from build123d import *

# Parameters (mm, degrees)
BOSS_EXTRUDE1_DEPTH = 9
SKETCH2_R           = 2.165
CUT_EXTRUDE1_DEPTH  = 32.81587654


with BuildPart() as part:
    # Sketch1 → Boss-Extrude1 (new body)
    with BuildSketch(Plane.XY):
        with BuildLine():
            Line((29, -13.075), (29, -9.075))
            Line((29, -9.075), (13.955285737, -9.075))
            ThreePointArc((13.955285737, -9.075), (0, 0.425), (-13.955285737, -9.075))
            Line((-13.955285737, -9.075), (-29, -9.075))
            Line((-29, -9.075), (-29, -13.075))
            Line((-29, -13.075), (-10.897247359, -13.075))
            ThreePointArc((-10.897247359, -13.075), (0, -3.575), (10.897247359, -13.075))
            Line((10.897247359, -13.075), (29, -13.075))
        make_face()
    extrude(amount=BOSS_EXTRUDE1_DEPTH)

    # Sketch2 → Cut-Extrude1 (cut, through all)
    with BuildSketch(Plane(origin=(0, -9.075, 0), x_dir=(1, 0, 0), z_dir=(0, 1, 0))):
        with Locations(Location((-23.50000005, -4.5, 0), (0, 0, 180))):
            Circle(SKETCH2_R)
        with Locations(Location((23.50000005, -4.5, 0), (0, 0, 180))):
            Circle(SKETCH2_R)
    extrude(amount=-CUT_EXTRUDE1_DEPTH, mode=Mode.SUBTRACT)


solid = part.part
Read the model definition and answer for the solid it produces. Units are mm, in the model's axes. A direction names the side the tool comes from. Coordinates: 2 decimals unless noted, no trailing zeros. Loops run counter-clockwise (first coordinate to the right, second up) from the corner with the lowest first, then second, coordinate; pieces in that order, holes last. Notation, with made-up numbers: (69.5, 38) -> (110.5, 38) arc R16 cw to (110.5, 42) -> close; hole circle Ø5 at (1, -21.75). An arc over 180 degrees is marked (long way). Write item = value, one per line. Start each with the question number.
1) Given P1, Ø4.5, axis at x = 23, z = 5.5, coming from the +Y side (3 decimals); P2, Ø2, axis at x = -1.5, z = 7, coming from the -Y side; P3, Ø5, axis at x = 2, z = 6, coming from the +Y side (3 decimals); P4, Ø1.5, axis at x = -17.5, y = -8, coming from the -Z side, each flat-ended and moving along its own axis, determine where each tip first touches the part or whether it passes through.
2) The part is cut by section A-A, the plane z = 4.5. Determine the outline of the cut face in (x, y) (3 decimals).
3) The part is cut by section C-C, the plane y = -11. Determine the outline of the cut face in (x, z) (3 decimals).
4) For faces 1 (the face through (-20, -13.075, 4)), 2 (the face through (20, -9.075, 4)), 3 (the face through (-21, -9.075, 5)), determine the directions among +Z, -Z, +X, -X, +Y, -Y from which every point of the face is accessible in a straight line to the end or side of a thin tool.
5) Find the intervals of material crossed by L1, parallel to Z at x = -23.5, y = -10.65 (3 decimals); L2, parallel to Y at x = -14, z = 5.5 (3 decimals); L3, parallel to X at y = -6.5, z = 3.25, in increasing order. Write a range as from..to.
6) The part is cut by section B-B, the plane x = -23.5. Determine the outline of the cut face in (y, z) (3 decimals), plus the area to 3 significant figures.
7) The mould has two halves that part along X. Classify faces 4 (the face through (25.663, -11.047, 4.595)), 5 (the face through (0, -3, 0)), 6 (the face through (-21.337, -11.047, 4.595)), 7 (the face through (0.251, 0.423, 4.437)): pulls with the +X half, pulls with the -X half, needs draft (parallel to the pull), parting line crosses it, or undercut.
8) The part is cut by section D-D, the plane z = 8.25. Determine the outline of the cut face in (x, y) (3 decimals), plus the area to 3 significant figures.
Result:
q1.P1 = -9.075
q1.P2 = -3.86
q1.P3 = 0.425
q1.P4 = through
q2.outline = (-29, -13.075) -> (-25.665, -13.075) -> (-25.665, -9.075) -> (-29, -9.075) -> close; (-21.335, -13.075) -> (-10.897, -13.075) arc R11 cw to (10.897, -13.075) -> (21.335, -13.075) -> (21.335, -9.075) -> (13.955, -9.075) arc R15 ccw to (-13.955, -9.075) -> (-21.335, -9.075) -> close; (25.665, -13.075) -> (29, -13.075) -> (29, -9.075) -> (25.665, -9.075) -> close
q3.outline = (-29, 0) -> (-10.403, 0) -> (-10.403, 9) -> (-29, 9) -> close; (10.403, 0) -> (29, 0) -> (29, 9) -> (10.403, 9) -> close; hole circle Ø4.33 at (-23.5, 4.5); hole circle Ø4.33 at (23.5, 4.5)
q4.face_1 = +Z, -Z, +X, -X, -Y
q4.face_2 = +Z, -Z, +X, +Y
q4.face_3 = +Z, -Z, -X, +Y
q5.L1 = 0..2.335, 6.665..9
q5.L2 = -13.075..-9.075
q5.L3 = -12.64..-7.47, 7.47..12.64
q6.outline = (-13.075, 0) -> (-9.075, 0) -> (-9.075, 2.335) -> (-13.075, 2.335) -> close; (-13.075, 6.665) -> (-9.075, 6.665) -> (-9.075, 9) -> (-13.075, 9) -> close
q6.area = 18.7 mm²
q7.face_4 = undercut
q7.face_5 = needs draft
q7.face_6 = undercut
q7.face_7 = parting line crosses it
q8.outline = (-29, -13.075) -> (-10.897, -13.075) arc R11 cw to (10.897, -13.075) -> (29, -13.075) -> (29, -9.075) -> (13.955, -9.075) arc R15 ccw to (-13.955, -9.075) -> (-29, -9.075) -> close
q8.area = 267 mm²
